Autodesk Inventor part; units mm, degrees
ref_plane "Work Plane1" through (0, 0, -15) normal (0, 0, 1) x (1, 0, 0)
ref_plane "YZ Plane" through (0, 0, 0) normal (1, 0, 0) x (0, 1, 0)
ref_plane "XZ Plane" through (0, 0, 0) normal (0, 1, 0) x (-1, 0, 0)
sketch "Sketch1" plane through (0, 0, 0) normal (0, 0, 1) x (1, 0, 0)
  line L0 (0, 0) -> (25, 0)
  line L1 (25, 0) -> (25, 40)
  line L2 (25, 40) -> (0, 40)
  line L3 (0, 40) -> (0, 0)
  dimension "d1" = 25
  dimension "d2" = 40
  dimension "d3" = 25
extrude "Extrusion1" add sketch "Sketch1" against normal blind 30
sketch "Sketch2" plane through (25, 0, 0) normal (1, 0, 0) x (0, 0, -1)
  line L0 (0, 0) -> (30, 0)
  circle A0 centre (15, 6.56) radius 2.46
extrude "Extrusion2" cut sketch "Sketch2" against normal blind 30
sketch "Sketch3" plane through (0, 0, 0) normal (-1, 0, 0) x (0, 0, 1)
  line L0 (0, 0) -> (-30, 0)
  line L1 (-25.05, 0) -> (-4.95, 0)
  line L2 (-4.95, 0) -> (-4.95, 33.12)
  line L3 (-4.95, 33.12) -> (-25.05, 33.12)
  line L4 (-25.05, 33.12) -> (-25.05, 0)
  dimension "d11" = 20.1
extrude "Extrusion3" cut sketch "Sketch3" against normal blind 20
sketch "Sketch4" plane through (0, 0, 0) normal (0, -1, 0) x (1, 0, 0)
  line L0 (20, -4.95) -> (20, -25.05)
  line L1 (20, -15) -> (25, -15)
  line L2 (25, 0) -> (25, -30)
  line L3 (20, -8.025) -> (25, -8.025)
  line L4 (25, -8.025) -> (25, -21.975)
  line L5 (25, -21.975) -> (20, -21.975)
  line L6 (20, -21.975) -> (20, -8.025)
  line L7 (20, -8.025) -> (25, -21.975) construction
  line L8 (25, -8.025) -> (20, -21.975) construction
  line L9 (25, -12.54) -> (25, -17.46)
  point P0 (0, 0)
  point P1 (22.5, -15)
  dimension "d14" = 13.95
extrude "Extrusion4" add sketch "Sketch4" along normal blind 15
sketch "Sketch5" plane through (20, 0, 0) normal (-1, 0, 0) x (0, 0, 1)
  circle A0 centre (-15, 6.56) radius 2.46
  circle A1 centre (-15, 6.56) radius 4.7025
  circle A2 centre (-15, 6.56) radius 2.46
  circle A3 centre (-15, 6.56) radius 2.46
  point P0 (0, 0)
  dimension "d17" = 9.405
extrude "Extrusion5" cut sketch "Sketch5" against normal blind 2.1
sketch "Sketch6" plane through (25, 0, 0) normal (1, 0, 0) x (0, 0, -1)
  circle A0 centre (15, 6.56) radius 4.7025
  line L0 (15, 6.56) -> (15, 23.56)
  circle A1 centre (15, 23.56) radius 2.46
  point P0 (0, 0)
  dimension "d20" = 17
  dimension "d21" = 4.92
extrude "Extrusion6" cut sketch "Sketch6" against normal blind 10 contours A1
sketch "Sketch7" plane through (20, 0, 0) normal (-1, 0, 0) x (0, 0, 1)
  circle A0 centre (-15, 23.56) radius 2.46
  circle A1 centre (-15, 23.56) radius 4.7025
  point P0 (0, 0)
  dimension "d24" = 9.405
extrude "Extrusion7" cut sketch "Sketch7" against normal blind 2.1
sketch "Sketch9" plane through (25, 0, 0) normal (1, 0, 0) x (0, 0, -1)
  circle A0 centre (15, 6.56) radius 2.46
  circle A1 centre (15, 6.56) radius 2.46
  circle A2 centre (15, 23.56) radius 2.46
  circle A3 centre (15, 23.56) radius 2.46
  line L0 (30, 40) -> (30, 0)
  line L1 (30, 0) -> (30, 40)
  line L2 (30, 40) -> (0, 40)
  line L3 (0, 40) -> (0, 0)
  line L4 (0, 0) -> (8.025, 0)
  line L5 (21.975, 0) -> (21.975, -15)
  line L6 (21.975, -15) -> (8.025, -15)
  line L7 (8.025, -15) -> (8.025, 0)
  line L8 (0, 0) -> (8.025, 0)
  line L9 (21.975, 0) -> (30, 0)
extrude "Extrusion8" add sketch "Sketch9" along normal blind 5
sketch "Sketch10" plane through (0, 40, 0) normal (0, 1, 0) x (1, 0, 0)
  line L0 (0, 30) -> (30, 30)
  line L1 (30, 0) -> (0, 0)
  line L2 (0, 30) -> (30, 30)
  line L3 (30, 30) -> (30, 0)
  line L4 (30, 0) -> (0, 0)
  line L5 (0, 0) -> (0, 30)
extrude "Extrusion9" add sketch "Sketch10" along normal blind 30
sketch "Sketch12" plane through (30, 0, 0) normal (1, 0, 0) x (0, 0, -1)
  circle A0 centre (15, 6.56) radius 2.46
  line L0 (15, 6.56) -> (15, 15.06)
  circle A1 centre (15, 15.06) radius 2.525
  point P0 (0, 0)
  dimension "d31" = 8.5
  dimension "d33" = 5.05
extrude "Extrusion10" cut sketch "Sketch12" against normal blind 30 contours A1
sketch "Sketch14" plane through (0, 0, 0) normal (0, 0, 1) x (1, 0, 0)
  line L0 (30, 70) -> (0, 70)
  line L1 (0, 70) -> (0, 85)
  line L2 (-15, 100) -> (-23, 100)
  line L3 (30, 100) -> (15, 115)
  line L4 (-23, 115) -> (15, 115)
  line L5 (30, 0) -> (30, 70)
  line L6 (30, 100) -> (30, 70)
  line L7 (-20.5, 113.5) -> (-23, 115)
  line L8 (-20.5, 101.5) -> (-23, 100)
  line L9 (-18, 107.5) -> (-20.5, 101.5)
  line L10 (-18, 107.5) -> (-20.5, 113.5)
  arc A0 (0, 85) -> (-15, 100) centre (-15, 85) ccw
  point P0 (0, 0)
  point P1 (0, 100)
  dimension "d47" = 30
  dimension "d49" = 15
  dimension "d54" = 15
extrude "Extrusion12" add sketch "Sketch14" against normal blind 30
sketch "Sketch15" plane through (0, 0, -25.05) normal (-1, 0, 0) x (0, 0, 1)
  line L0 (0, 33.12) -> (20.1, 33.12)
  line L1 (20.1, 33.12) -> (20.1, 0)
  line L2 (0, 33.12) -> (20.1, 33.12)
  line L3 (20.1, 33.12) -> (20.1, 31.1)
  line L4 (20.1, 31.1) -> (0, 31.1)
  line L5 (0, 31.1) -> (0, 33.12)
  point P0 (25.05, 0)
  dimension "d57" = 2.02
extrude "Extrusion13" add sketch "Sketch15" against normal blind 20
sketch "Sketch17" plane through (0, 0, 0) normal (0, 0, 1) x (1, 0, 0)
  line L0 (-23, 115) -> (15, 115)
  line L1 (-23, 115) -> (15, 115)
  line L2 (30, 0) -> (30, 100)
  line L3 (15, 115) -> (30, 100)
  line L4 (30, 100) -> (30, 85)
  arc A0 (0, 85) -> (-15, 100) centre (-15, 85) ccw
  line L5 (30, 85) -> (0, 85)
  arc A1 (0, 85) -> (-15, 100) centre (-15, 85) ccw
  line L6 (-15, 100) -> (-23, 100)
  line L7 (-15, 100) -> (-23, 100)
  line L8 (-23, 100) -> (-20.5, 101.5)
  line L9 (-23, 100) -> (-20.5, 101.5)
  line L10 (-20.5, 101.5) -> (-18, 107.5)
  line L11 (-20.5, 101.5) -> (-18, 107.5)
  line L12 (-18, 107.5) -> (-20.5, 113.5)
  line L13 (-18, 107.5) -> (-20.5, 113.5)
  line L14 (-20.5, 113.5) -> (-23, 115)
  point P0 (0, 0)
extrude "Extrusion14" add sketch "Sketch17" along normal blind 45
ref_plane "Work Plane1" through (0, 0, -15) normal (0, 0, 1) x (1, 0, 0)
mirror "Mirror1" about plane through (0, 0, -15) normal (0, 0, 1) of "Extrusion14"
properties part number "12mm_x_120mm"
Here's how the part is built. I have some questions about the finished solid (model axes, mm). A direction names the side the tool comes from. Round coordinates to 2 decimals unless told otherwise and drop trailing zeros. Loops run counter-clockwise (first coordinate to the right, second up) from the corner with the lowest first, then second, coordinate; pieces in that order, holes last. Notation, with made-up numbers: (54.5, 4) -> (72.5, 4) arc R27 ccw to (72.5, 39) -> close; hole circle Ø2 at (-9.75, 7.5). An arc over 180 degrees is marked (long way). Answer as CSV lines item,"result".
1. If we section it at B-B on z = -15: Count the separate pieces of the cut face and the enclosed holes in it, plus the area to 3 significant figures.
Final values:
separate pieces,"4"
enclosed holes,"0"
area,"3,040 mm^2"
2. If we section it at A-A on y = 15.06: Please give me the cut outline in (x, z) (3 decimals).
Final values:
outline,"(0, -30) -> (30, -30) -> (30, -17.525) -> (20, -17.525) -> (20, -25.05) -> (0, -25.05) -> close; (0, -4.95) -> (20, -4.95) -> (20, -12.475) -> (30, -12.475) -> (30, 0) -> (0, 0) -> close"
3. If we section it at D-D on z = 19.5: Please give me the cut outline in (x, y), plus the area to 3 significant figures.
Final values:
outline,"(-23, 100) -> (-15, 100) arc R15 cw to (0, 85) -> (30, 85) -> (30, 100) -> (15, 115) -> (-23, 115) -> (-20.5, 113.5) -> (-18, 107.5) -> (-20.5, 101.5) -> close"
area,"1,130 mm^2"
4. For pin 1 (5.5 mm diameter, centred on y = 6.56, z = -15, fed in from -X); pin 2 (7.5 mm diameter, centred on y = 23.56, z = -15, fed in from +X); pin 3 (10 mm diameter, centred on x = 9, z = 8, fed in from -Y); pin 4 (8 mm diameter, centred on x = -14.5, z = -34, fed in from -Y), each with a flat end and sliding along its axis, tell me the tip position at first contact or that it passes through.
Final values:
pin 1,"stops at x = 22.1"
pin 2,"stops at x = 30"
pin 3,"stops at y = 85"
pin 4,"stops at y = 99.31"
5. Which directions (+Z, -Z, +X, -X, +Y, -Y) give clear straight access to the entire face, cutting with the end or side of a thin tool? Please do faces 4 (the face through (25, -7, -21.975)), 5 (the face through (-19.268, 110.542, -14.16)), 6 (the face through (10, 15, -4.95)).
Final values:
face 4,"-Z, +X, -X, -Y"
face 5,"+Z, -Z, -X"
face 6,"-X, -Y"
6. If I drill on L1, parallel to Y at x = 28, z = -15 (3 decimals); L2, parallel to Z at x = 24, y = 23.56; L3, parallel to Z at x = 21, y = 6, over which ranges is the centre line in solid material (lowest first)?
Final values:
L1,"y = -15 to 4.1, 9.02 to 12.535, 17.585 to 21.1, 26.02 to 102"
L2,"z = -30 to -17.46, -12.54 to 0"
L3,"z = -30 to -19.67, -10.33 to 0"
7. Thinking about a two-plate mould opening in Z: for faces 1 (the face through (21.035, 27.525, -12.472)), 2 (the face through (4, 100, -75)), 3 (the face through (-19.232, 104.542, -14.16)), which applies, released by +Z, released by -Z, zero draft, split by the parting line, or undercut?
Final values:
face 1,"undercut"
face 2,"released by -Z"
face 3,"zero draft"
8. If we section it at C-C on x = 26: Please give me the cut outline in (y, z) (3 decimals).
Final values:
outline,"(-15, -21.975) -> (0, -21.975) -> (0, -30) -> (85, -30) -> (85, -75) -> (104, -75) -> (104, 45) -> (85, 45) -> (85, 0) -> (0, 0) -> (0, -8.025) -> (-15, -8.025) -> close; hole circle Ø4.92 at (6.56, -15); hole circle Ø5.05 at (15.06, -15); hole circle Ø4.92 at (23.56, -15)"
